from build123d import *

# Parameters (mm, degrees)
F0_W      = 20
F0_H      = 5
F1_DEPTH  = 2
F2_W      = 16
F2_H      = 2
F3_DEPTH  = 7
F5_DEPTH  = 2
F6_W      = 25.4
F6_H      = 6
F7_DEPTH  = 1.5
F8_W      = 1
F8_H      = 6
F9_DEPTH  = 7.5
F10_W     = 1
F10_H     = 2.5
F11_DEPTH = 23.4


with BuildPart() as f1:
    # F0 (on Front) → F1 (new body)
    with BuildSketch(Plane.XZ):
        Rectangle(F0_W, F0_H)
    extrude(amount=F1_DEPTH)

    # F2 (on face) → F3 (join)
    with BuildSketch(Plane.XZ.offset(2)):
        Rectangle(F2_W, F2_H)
    extrude(amount=F3_DEPTH)

    # F4 (on face) → F5 (join, through all)
    with BuildSketch(Plane.XY.offset(1)):
        Polygon((12.7, -14), (8, -9), (-8, -9), (-12.7, -14), align=None)
    extrude(amount=-F5_DEPTH)

    # F6 (on face) → F7 (join)
    with BuildSketch(Plane.XZ.offset(14)):
        Rectangle(F6_W, F6_H)
    extrude(amount=F7_DEPTH)

    # F8 (on face) → F9 (join)
    with BuildSketch(Plane.XZ.offset(15.5)):
        with Locations((-12.2, 0)):
            Rectangle(F8_W, F8_H)
        with Locations((12.2, 0)):
            Rectangle(F8_W, F8_H)
    extrude(amount=F9_DEPTH)

    # F10 (on face) → F11 (join, through all)
    with BuildSketch(Plane.YZ.offset(-11.7)):
        with Locations((-22, 1.25)):
            Rectangle(F10_W, F10_H)
    extrude(amount=F11_DEPTH)


solid = f1.part
Build history of the part. All positions in model axes, mm. A direction names the side the tool comes from. Round coordinates to 2 decimals unless told otherwise and drop trailing zeros. Loops run counter-clockwise (first coordinate to the right, second up) from the corner with the lowest first, then second, coordinate; pieces in that order, holes last. Notation, with made-up numbers: (-36, 7) -> (2, 7) arc R33 ccw to (2, 45) -> close; hole circle Ø8 at (20, 71.25). An arc over 180 degrees is marked (long way). One line per item, written item: value. Start each with the question number.
Q1. Two-plate mould, pull along X, no slides. Class faces 1 (the face through (0, -21.5, 1)), 2 (the face through (0, -15, -3)), 3 (the face through (-12.7, -18, 0)): released by +X, released by -X, zero draft, split by the parting line, or undercut.
Q2. Cut at A-A on z = 1.95. List the corners of the cut face in (x, y).
Q3. Cut at C-C on y = -16.75. List the corners of the cut face in (x, z), plus the area to 3 significant figures.
Q4. Cut at D-D on z = -1.95. List the corners of the cut face in (x, y).
Q5. Cut at B-B on x = -5.25. List the corners of the cut face in (y, z), plus the area to 3 significant figures.
Q6. 3-axis set-ups, long thin cutter, end or side, ignore diameter. For faces 4 (the face through (0, -15.5, 0)), 5 (the face through (0, -1, 2.5)), 6 (the face through (0, -8, -1)), 7 (the face through (-10.317, -11.465, 0.014)), 8 (the face through (0, -8, 1)): which of +Z, -Z, +X, -X, +Y, -Y reach the whole face in a straight line?
Q7. Probe line 1 along Y through (x, z) = (-3.75, 2.15); line 2 along X through (y, z) = (-16, -0.55); line 3 along Y through (x, z) = (9, -2.3). List the from-to ranges inside material, lowest first.
Q8. Drop flat-ended pins along their axis: pin 1 Ø1.5 at (x, y) = (-6, -7.5) entering from +Z; pin 2 Ø2.5 at (x, z) = (1, -1) entering from -Y; pin 3 Ø1.6 at (y, z) = (-4.5, 0) entering from -X. Give the stop position or say it passes through.
Computed:
1. face 1: undercut
1. face 2: zero draft
1. face 3: released by -X
2. outline: (-12.7, -23) -> (-11.7, -23) -> (-11.7, -22.5) -> (11.7, -22.5) -> (11.7, -23) -> (12.7, -23) -> (12.7, -14) -> (-12.7, -14) -> close; (-10, -2) -> (10, -2) -> (10, 0) -> (-10, 0) -> close; hole (-11.7, -21.5) -> (11.7, -21.5) -> (11.7, -15.5) -> (-11.7, -15.5) -> close
3. outline: (-12.7, -3) -> (-11.7, -3) -> (-11.7, 3) -> (-12.7, 3) -> close; (11.7, -3) -> (12.7, -3) -> (12.7, 3) -> (11.7, 3) -> close
3. area: 12.0 mm²
4. outline: (-12.7, -23) -> (-11.7, -23) -> (-11.7, -15.5) -> (11.7, -15.5) -> (11.7, -23) -> (12.7, -23) -> (12.7, -14) -> (-12.7, -14) -> close; (-10, -2) -> (10, -2) -> (10, 0) -> (-10, 0) -> close
5. outline: (-22.5, 0) -> (-21.5, 0) -> (-21.5, 2.5) -> (-22.5, 2.5) -> close; (-15.5, -3) -> (-14, -3) -> (-14, -1) -> (-2, -1) -> (-2, -2.5) -> (0, -2.5) -> (0, 2.5) -> (-2, 2.5) -> (-2, 1) -> (-14, 1) -> (-14, 3) -> (-15.5, 3) -> close
5. area: 45.5 mm²
6. face 4: +Z, -Z
6. face 5: +Z, +X, -X, +Y
6. face 6: -Z, +X, -X
6. face 7: +Z, -Z, -X
6. face 8: +Z, +X, -X
7. line 1: -22.5 to -21.5, -15.5 to -14, -2 to 0
7. line 2: -12.7 to -11.7, 11.7 to 12.7
7. line 3: -15.5 to -14, -2 to 0
8. pin 1: z = 1
8. pin 2: y = -22.5
8. pin 3: x = -8
